from build123d import *

# Parameters (mm, degrees)
EXTRUDE_1_DEPTH     = 5
SKETCH_2_R          = 1.25
CUT_EXTRUDE_1_DEPTH = 5


with BuildPart() as part:
    # 草图1 → 凸台-拉伸1 (new body)
    with BuildSketch(Plane(origin=(0, 0, 0), x_dir=(1, 0, 0), z_dir=(0, 1, 0))):
        with BuildLine():
            Line((0, 0), (5, 0))
            ThreePointArc((5, 0), (8.5, 1.5), (12, 0))
            Line((12, 0), (12.212191433, 0.212191433))
            ThreePointArc((12.212191433, 0.212191433), (8.561418456, 1.799632562), (4.873707127, 0.3))
            Line((4.873707127, 0.3), (0, 0.3))
            Line((0, 0.3), (0, 0))
        make_face()
    extrude(amount=EXTRUDE_1_DEPTH)

    # 草图2 → 切除-拉伸1 (cut)
    with BuildSketch(Plane(origin=(0, 0, -0.3), x_dir=(-1, 0, 0), z_dir=(0, 0, -1))):
        with Locations((-2.5, 2.5)):
            Circle(SKETCH_2_R)
    extrude(amount=-CUT_EXTRUDE_1_DEPTH, mode=Mode.SUBTRACT)


solid = part.part
Model file for the job. Use its own axes, mm. Round coordinates to 2 decimals unless told otherwise and drop trailing zeros. Loops run counter-clockwise (first coordinate to the right, second up) from the corner with the lowest first, then second, coordinate; pieces in that order, holes last.
1. Band-saw the part on C-C, the plane y = 2.5. List the corners of the cut face in (x, z).
Check values:
outline: (0, -0.3) - (1.25, -0.3) - (1.25, 0) - (0, 0) - close; (3.75, -0.3) - (4.87, -0.3) arc R5.13 ccw to (12.21, -0.21) - (12, 0) arc R4.83 cw to (5, 0) - (3.75, 0) - close
2. Mould opens along X. For faces 1 (the cylindrical face through (1.31, 2.88, -0.15)), 2 (the flat face through (2, 1, 0)), 3 (the cylindrical face through (8.6, 2.5, -1.8)), 4 (the cylindrical face through (8.4, 2.5, -1.5)) say: +X half, -X half, draft (parallel to the pull), parting line (faces both ways), or undercut.
Check values:
face 1: undercut
face 2: draft
face 3: parting line
face 4: undercut
3. Band-saw the part on B-B, the plane x = 2.5. List the corners of the cut face in (y, z), and give its area (3 significant figures).
Check values:
outline: (0, -0.3) - (1.25, -0.3) - (1.25, 0) - (0, 0) - close; (3.75, -0.3) - (5, -0.3) - (5, 0) - (3.75, 0) - close
area: 0.750 mm2
4. Band-saw the part on D-D, the plane y = 3.3. List the corners of the cut face in (x, z).
Check values:
outline: (0, -0.3) - (1.54, -0.3) - (1.54, 0) - (0, 0) - close; (3.46, -0.3) - (4.87, -0.3) arc R5.13 ccw to (12.21, -0.21) - (12, 0) arc R4.83 cw to (5, 0) - (3.46, 0) - close
5. Wall check: probe 1 along Y at (x, z) = (2.5, -0.2); probe 2 along Z at (x, y) = (1.75, 1.35); probe 3 along X at (y, z) = (3.05, -0.45). Give the ranges that are in metal, low to high.
Check values:
probe 1: y = 0 to 1.25, 3.75 to 5
probe 2: z = -0.3 to 0
probe 3: x = 5.03 to 5.49, 11.51 to 11.97
6. Band-saw the part on A-A, the plane z = -0.45. List the corners of the cut face in (x, y).
Check values:
outline: (5.03, 0) - (5.49, 0) - (5.49, 5) - (5.03, 5) - close; (11.51, 0) - (11.97, 0) - (11.97, 5) - (11.51, 5) - close
7. Drop flat-ended pins along their axis: P1, Ø1.5, axis at x = 6.5, y = 3, coming from the +Z side; P2, Ø1.5, axis at x = 7.5, y = 2, coming from the +Z side; P3, Ø2, axis at x = 2.5, y = 2.5, coming from the +Z side; P4, Ø2, axis at x = 4, y = 4, coming from the -Z side. Give the stop position or say it passes through.
Check values:
P1: stops at z = -0.64
P2: stops at z = -1.17
P3: passes through
P4: stops at z = -0.42
